from build123d import *

# Parameters (mm, degrees)
SKETCH_1_R            = 3
EXTRUDE_251_DEPTH     = 2.5
CHAMFER_1_SIZE        = 1.5
CUT_EXTRUDE_459_DEPTH = 1.3
SKETCH_3_R            = 1.5
EXTRUDE_571_DEPTH     = 10


with BuildPart() as part:
    # 草图1 → Extrude 251 (new body)
    with BuildSketch(Plane(origin=(0, 0, 0), x_dir=(1, 0, 0), z_dir=(0, 1, 0))):
        Circle(SKETCH_1_R)
    extrude(amount=EXTRUDE_251_DEPTH)

    # 倒角1
    chamfer_1_edges = [part.edges().sort_by_distance(p)[0] for p in [
        (-3, 0, 0),
    ]]
    chamfer(chamfer_1_edges, length=CHAMFER_1_SIZE)

    # 草图2 → Cut-Extrude 459 (cut)
    with BuildSketch(Plane(origin=(0, 2.5, 0), x_dir=(1, 0, 0), z_dir=(0, 1, 0))):
        Polygon((1.443375673, 0), (0.721687836, 1.25), (-0.721687836, 1.25), (-1.443375673, 0), (-0.721687836, -1.25), (0.721687836, -1.25), align=None)
    extrude(amount=-CUT_EXTRUDE_459_DEPTH, mode=Mode.SUBTRACT)

    # 草图3 → Extrude 571 (add)
    with BuildSketch(Plane.XZ):
        Circle(SKETCH_3_R)
    extrude(amount=EXTRUDE_571_DEPTH)


solid = part.part
The listing builds one solid part. Answer for the finished solid, in the listing's coordinates (mm). A direction names the side the tool comes from. Coordinates: 2 decimals unless noted, no trailing zeros. Order: outer loops, then holes, each group sorted by start corner. A loop starts at its lowest first (then second) coordinate and runs counter-clockwise, first axis right, second up. Notation, with made-up numbers: M 50.25,58.5 L 84.25,58.5 A28 cw 84.25,94.5 Z; hole C 33.5,51.5 d9. An arc over 180 degrees is marked long. Use CSV: the item, a comma, the result in double quotes.
Q1. Section C-C (y = 0.5) is taken. Determine the outline of the cut face in (x, z).
Here are the results:
outline,"C 0,0 d4"
Q2. A tool of negligible diameter and unlimited length cuts with its end or side. For faces 4 (the flat face through (0, -10, 0)), 5 (the flat face through (1.08, 1.86, 0.63)), from which of +Z, -Z, +X, -X, +Y, -Y can it reach the whole face along a straight path? Write none if from no direction.
Here are the results:
face 4,"+Z, -Z, +X, -X, -Y"
face 5,"+Y"
Q3. Straight lines are drawn through the part: L1, parallel to Y at x = -0.05, z = -1; L2, parallel to X at y = -1.5, z = -0.4; L3, parallel to Y at x = -2, z = 2. For each, find the intervals that lie inside material, in ascending order.
Here are the results:
L1,"-10 to 1.2"
L2,"-1.45 to 1.45"
L3,"1.33 to 2.5"
Q4. Section B-B (y = -1.5) is taken. Determine the outline of the cut face in (x, z).
Here are the results:
outline,"C 0,0 d3"
Q5. Determine the mould class of faces 1 (the flat face through (1.3, 2.5, 0.6)), 2 (the cylindrical face through (-1.5, -4.93, 0.07)), 3 (the flat face through (0, 2, -1.25)) for opening direction Z: pulls with the +Z half, pulls with the -Z half, needs draft (parallel to the pull), parting line crosses it, or undercut.
Here are the results:
face 1,"needs draft"
face 2,"parting line crosses it"
face 3,"undercut"
Q6. Section A-A (x = 0) is taken. Determine the outline of the cut face in (y, z).
Here are the results:
outline,"M -10,-1.5 L 0,-1.5 L 1.5,-3 L 2.5,-3 L 2.5,-1.25 L 1.2,-1.25 L 1.2,1.25 L 2.5,1.25 L 2.5,3 L 1.5,3 L 0,1.5 L -10,1.5 Z"
Q7. Given pin 1 Ø0.8 at (x, z) = (0.5, -0.5) entering from +Y; pin 2 Ø1.5 at (y, z) = (-4, 0) entering from +X; pin 3 Ø3 at (x, y) = (0, -3) entering from +Z, each flat-ended and moving along its own axis, determine where each tip first touches the part or whether it passes through.
Here are the results:
pin 1,"y = 1.2"
pin 2,"x = 1.5"
pin 3,"z = 1.5"
